Can you work these out from the model? Positions are in its coordinate system, mm. A direction names the side the tool comes from. Give positions to 0.01 mm unless a question says otherwise; leave off trailing zeros. Write each loop counter-clockwise with the first axis right and the second up, starting at its lowest first coordinate (ties: lowest second). Pieces come first, ordered by that corner, then holes. Notation, with made-up numbers: (0.5, -16) -> (50.5, -16) arc R19 ccw to (50.5, -6) -> close; hole circle Ø2 at (-19, 32.25). An arc over 180 degrees is marked (long way). Answer as CSV lines item,"result". Start each with the question number.
1. If we section it at C-C on y = -11: Write out the boundary of the cut face in (x, z).
2. If we mould it in two halves opening along X, with no side actions, what happens to faces 1 (the face through (17.323, 1, -48)), 2 (the face through (-21.009, -40.744, 19.265)), 3 (the face through (-17.323, 1, -49))? For each: pulls with the +X half, pulls with the -X half, needs draft (parallel to the pull), parting line crosses it, or undercut.
3. If we section it at B-B on x = 0: Write out the boundary of the cut face in (y, z).
4. If we section it at A-A on y = 15: Write out the boundary of the cut face in (x, z).
5. I'm going to push flat-ended pins straight in: P1, Ø15.5, axis at y = -25, z = -50, coming from the -X side; P2, Ø1.5, axis at x = -37.5, y = 12, coming from the -Z side; P3, Ø4, axis at x = -51.5, y = 21, coming from the +Z side. Where does each tip first touch, or does it pass through?
6. I need wall thicknesses on line 1 (Z direction, x = 46, y = 45.5); line 2 (Y direction, x = -3, z = -16.5); line 3 (X direction, y = 4.5, z = 47.5). Which ranges of each line are inside material? Lowest first, please. Write a range as [from, to].
7. On a 3-axis mill with a long thin cutter (end or side, diameter ignored), from which of +Z, -Z, +X, -X, +Y, -Y can I reach the whole of each face in a straight line? I mean faces 4 (the face through (31.22, 25.76, 33.92)), 5 (the face through (-33.64, 25.76, -31.52)), 6 (the face through (-31.446, -25.756, 33.71)). Say none if no direction works.
```python
from build123d import *

# Parameters (mm, degrees)
F0_R     = 44.7502434254
F1_DEPTH = 50.8
F1_TAPER = -3
F2_W     = 24.901330471
F2_H     = 27.4275690317
F2_W_2   = 37.1715724468
F2_H_2   = 29.9537181854
F2_W_3   = 11.5484520793
F2_H_3   = 1.9849091768
F3_DEPTH = 101.6
F4_R     = 27.9776430022
F5_DEPTH = 25.4
F5_TAPER = -3


with BuildPart() as f1:
    # F0 (on Front) → F1 (new body, symmetric)
    with BuildSketch(Plane.XZ):
        Circle(F0_R)
    extrude(amount=F1_DEPTH, both=True, taper=F1_TAPER)

    # F2 (on face) → F3 (join)
    with BuildSketch(Plane(origin=(0, 50.8, 0), x_dir=(-1, 0, 0), z_dir=(0, 1, 0))):
        with BuildLine():
            ThreePointArc((47.412558613, 0), (46.8017179006, 7.5861660792), (44.9849353222, 14.9768590927))
            Line((44.9849353222, 14.9768590927), (17.8640037775, 14.9768590927))
            Line((17.8640037775, 14.9768590927), (17.8640037775, -14.9768590927))
            Line((17.8640037775, -14.9768590927), (44.9849353222, -14.9768590927))
            ThreePointArc((44.9849353222, -14.9768590927), (46.8017179006, -7.5861660792), (47.412558613, 0))
        make_face()
        with Locations((0, 40.0586426258)):
            Rectangle(F2_W, F2_H)
        with Locations((36.4497900009, 0)):
            Rectangle(F2_W_2, F2_H_2)
        Polygon((-17.3226743937, -55.5769503117), (17.3226743937, -55.5769503117), (17.3226743937, -14.7964656353), (-5.7742223144, -14.7964656353), (-5.7742223144, -16.7813748121), (-17.3226743937, -16.7813748121), align=None)
        Polygon((-57.3813542724, -16.7813748121), (-17.3226743937, -16.7813748121), (-17.3226743937, -14.7964656353), (-5.7742223144, -14.7964656353), (-5.7742223144, 16.7813748121), (-57.3813542724, 16.7813748121), align=None)
        with Locations((-11.548448354, -15.7889202237)):
            Rectangle(F2_W_3, F2_H_3)
    extrude(amount=-F3_DEPTH)

    # F4 (on face) → F5 (cut)
    with BuildSketch(Plane.XZ.offset(50.8)):
        Circle(F4_R)
    extrude(amount=-F5_DEPTH, taper=F5_TAPER, mode=Mode.SUBTRACT)


solid = f1.part
```
Computed values:
1,outline,"(-55.04, -14.98) -> (-42.78, -14.98) arc R45.33 ccw to (-17.32, -41.89) -> (-17.32, -55.58) -> (17.32, -55.58) -> (17.32, -41.89) arc R45.33 ccw to (42.11, -16.78) -> (57.38, -16.78) -> (57.38, 16.78) -> (42.11, 16.78) arc R45.33 ccw to (12.45, 43.58) -> (12.45, 53.77) -> (-12.45, 53.77) -> (-12.45, 43.58) arc R45.33 ccw to (-42.78, 14.98) -> (-55.04, 14.98) -> close"
2,face 1,"pulls with the +X half"
2,face 2,"undercut"
2,face 3,"pulls with the -X half"
3,outline,"(-50.8, -55.58) -> (50.8, -55.58) -> (50.8, 53.77) -> (-50.8, 53.77) -> (-50.8, 27.98) -> (-25.4, 29.31) -> (-25.4, -29.31) -> (-50.8, -27.98) -> close"
4,outline,"(-55.04, -14.98) -> (-43, -14.98) arc R45.54 ccw to (-17.32, -42.11) -> (-17.32, -55.58) -> (17.32, -55.58) -> (17.32, -42.11) arc R45.54 ccw to (42.33, -16.78) -> (57.38, -16.78) -> (57.38, 16.78) -> (42.33, 16.78) arc R45.54 ccw to (12.45, 43.8) -> (12.45, 53.77) -> (-12.45, 53.77) -> (-12.45, 43.8) arc R45.54 ccw to (-43, 14.98) -> (-55.04, 14.98) -> close"
5,P1,"stops at x = -18.37"
5,P2,"stops at z = -26.62"
5,P3,"stops at z = 14.98"
6,line 1,"z = [-16.78, 16.78]"
6,line 2,"y = [-25.4, 50.8]"
6,line 3,"x = [-12.45, 12.45]"
7,face 4,"+Z, +X"
7,face 5,"-Z, -X"
7,face 6,"+Z, -X"
